from build123d import *

# Parameters (mm, degrees)
SKETCH1_W           = 150
SKETCH1_H           = 75
SKETCH1_W_2         = 11
SKETCH1_H_2         = 22
BOSS_EXTRUDE1_DEPTH = 10
SKETCH2_W           = 10
SKETCH2_H           = 20
BOSS_EXTRUDE2_DEPTH = 4
SKETCH3_W           = 20
SKETCH3_H           = 3
BOSS_EXTRUDE3_DEPTH = 10
SKETCH4_W           = 20
SKETCH4_H           = 3
BOSS_EXTRUDE4_DEPTH = 5


with BuildPart() as part:
    # Sketch1 → Boss-Extrude1 (new body)
    with BuildSketch(Plane(origin=(0, 0, 0), x_dir=(0, 1, 0), z_dir=(0, 0, 1))):
        Rectangle(SKETCH1_W, SKETCH1_H)
        with Locations((-59.5, -11.5)):
            Rectangle(SKETCH1_W_2, SKETCH1_H_2, mode=Mode.SUBTRACT)
    extrude(amount=BOSS_EXTRUDE1_DEPTH)

    # Sketch2 → Boss-Extrude2 (add)
    with BuildSketch(Plane.XY.offset(10)):
        with Locations((12.5, 25)):
            Rectangle(SKETCH2_W, SKETCH2_H)
    extrude(amount=BOSS_EXTRUDE2_DEPTH)

    # Sketch3 → Boss-Extrude3 (add)
    with BuildSketch(Plane.YZ.offset(37.5)):
        with Locations((-45, 5)):
            Rectangle(SKETCH3_W, SKETCH3_H)
        with Locations((35, 5)):
            Rectangle(SKETCH3_W, SKETCH3_H)
    extrude(amount=BOSS_EXTRUDE3_DEPTH)

    # Sketch4 → Boss-Extrude4 (add)
    with BuildSketch(Plane(origin=(0, 75, 0), x_dir=(-1, 0, 0), z_dir=(0, 1, 0))):
        with Locations((0, 5)):
            Rectangle(SKETCH4_W, SKETCH4_H)
    extrude(amount=BOSS_EXTRUDE4_DEPTH)


solid = part.part
Check sheet for the modelled part. Datum: model origin and axes. Units: mm. A direction names the side the tool comes from. Round coordinates to 2 decimals unless told otherwise and drop trailing zeros. Order: outer loops, then holes, each group sorted by start corner. A loop starts at its lowest first (then second) coordinate and runs counter-clockwise, first axis right, second up.
Q1. Scan lines: L1, parallel to Y at x = 21.5, z = 7.25; L2, parallel to Z at x = 21, y = -3; L3, parallel to X at y = 22, z = 7.75. Record each from-to range of solid material in increasing order.
Filled sheet:
L1: y = -75 to -65, -54 to 75
L2: z = 0 to 10
L3: x = -37.5 to 37.5
Q2. Cross-section at B-B, the plane y = -60. Enter the section's corners in (x, z), plus the area to 3 significant figures.
Filled sheet:
outline: (-37.5, 0) - (0.5, 0) - (0.5, 10) - (-37.5, 10) - close; (22.5, 0) - (37.5, 0) - (37.5, 10) - (22.5, 10) - close
area: 530 mm2
Q3. Cross-section at C-C, the plane z = 8. Enter the section's corners in (x, y).
Filled sheet:
outline: (-37.5, -75) - (37.5, -75) - (37.5, 75) - (-37.5, 75) - close; hole (0.5, -65) - (22.5, -65) - (22.5, -54) - (0.5, -54) - close
Q4. Cross-section at D-D, the plane x = 41. Enter the section's corners in (y, z), plus the area to 3 significant figures.
Filled sheet:
outline: (-55, 3.5) - (-35, 3.5) - (-35, 6.5) - (-55, 6.5) - close; (25, 3.5) - (45, 3.5) - (45, 6.5) - (25, 6.5) - close
area: 120 mm2
Q5. Cross-section at A-A, the plane x = 3.5. Enter the section's corners in (y, z).
Filled sheet:
outline: (-75, 0) - (-65, 0) - (-65, 10) - (-75, 10) - close; (-54, 0) - (75, 0) - (75, 3.5) - (80, 3.5) - (80, 6.5) - (75, 6.5) - (75, 10) - (-54, 10) - close
Q6. Draft check along X on faces 1 (the face through (1, 75, 3)), 2 (the face through (7.5, 25, 12)), 3 (the face through (12, -54, 5)). Enter one of: pulls with the +X half, pulls with the -X half, needs draft (parallel to the pull), parting line crosses it, or undercut.
Filled sheet:
face 1: needs draft
face 2: pulls with the -X half
face 3: undercut
Q7. Depth check by flat-ended pin: P1, Ø2.5, axis at x = 1, y = 78.5, coming from the +Z side; P2, Ø5, axis at x = 20, y = 7, coming from the +Z side; P3, Ø8, axis at x = 41, y = -45.5, coming from the -Z side; P4, Ø1.5, axis at y = 78, z = 5, coming from the -X side. Enter the tip coordinate at first touch or a pass-through.
Filled sheet:
P1: stops at z = 6.5
P2: stops at z = 10
P3: stops at z = 0
P4: stops at x = -10
Q8. Set-up check for faces 4 (the face through (42, -45, 6.5)), 5 (the face through (22.5, -60, 5)), 6 (the face through (42, 25, 5)), 7 (the face through (0, 77, 6.5)): record each of +Z, -Z, +X, -X, +Y, -Y from which the full face is reachable in a straight line by a thin tool's end or side.
Filled sheet:
face 4: +Z, +X, +Y, -Y
face 5: +Z, -Z
face 6: +Z, -Z, +X
face 7: +Z, +X, -X, +Y
